```python
from build123d import *

# Parameters (mm, degrees)
SKETCH_1_W          = 100
SKETCH_1_H          = 50
EXTRUDE_1_DEPTH     = 10
SKETCH_2_R          = 5
EXTRUDE_2_DEPTH     = 10
HOLE_WIZARD_1_D     = 8.647
HOLE_WIZARD_1_DEPTH = 26.2
HOLE_WIZARD_1_TIP   = 2.597820886
FILLET_3_R          = 1
CHAMFER_2_SIZE      = 1
CHAMFER_3_SIZE      = 0.5


with BuildPart() as part:
    # 草圖1 → 擠出1 (new body)
    with BuildSketch(Plane(origin=(0, 0, 0), x_dir=(-1, 0, 0), z_dir=(0, 1, 0))):
        Rectangle(SKETCH_1_W, SKETCH_1_H)
    extrude(amount=EXTRUDE_1_DEPTH)

    # 草圖2 → 擠出2 (cut)
    with BuildSketch(Plane(origin=(0, 10, 0), x_dir=(-1, 0, 0), z_dir=(0, 1, 0))):
        with Locations(Location((-30, -12.5, 0), (0, 0, 90))):
            Circle(SKETCH_2_R)
        with Locations(Location((-30, 12.5, 0), (0, 0, 90))):
            Circle(SKETCH_2_R)
    extrude(amount=-EXTRUDE_2_DEPTH, mode=Mode.SUBTRACT)

    # 孔1
    with Locations(Plane(origin=(0, 10, 0), x_dir=(1, 0, 0), z_dir=(0, 1, 0))):
        with Locations((-30, -12.5), (-30, 12.5)):
            Hole(HOLE_WIZARD_1_D / 2, depth=HOLE_WIZARD_1_DEPTH)
            with Locations((0, 0, -(HOLE_WIZARD_1_DEPTH + HOLE_WIZARD_1_TIP / 2))):  # 118° drill point
                Cone(0, HOLE_WIZARD_1_D / 2, HOLE_WIZARD_1_TIP, mode=Mode.SUBTRACT)

    # 圓角3
    fillet_3_edges = [part.edges().sort_by_distance(p)[0] for p in [
        (-50, 5, -25),
        (50, 5, -25),
        (50, 5, 25),
        (-50, 5, 25),
    ]]
    fillet(fillet_3_edges, radius=FILLET_3_R)

    # 倒角2
    chamfer_2_edges = [part.edges().sort_by_distance(p)[0] for p in [
        (0, 0, -25),
        (0, 10, -25),
        (-50, 0, 0),
        (50, 0, 0),
        (0, 0, 25),
        (-49.707106781, 0, 24.707106781),
        (-49.707106781, 0, -24.707106781),
        (49.707106781, 0, 24.707106781),
        (49.707106781, 0, -24.707106781),
        (50, 10, 0),
        (-50, 10, 0),
        (0, 10, 25),
        (-49.707106781, 10, 24.707106781),
        (-49.707106781, 10, -24.707106781),
        (49.707106781, 10, 24.707106781),
        (49.707106781, 10, -24.707106781),
    ]]
    chamfer(chamfer_2_edges, length=CHAMFER_2_SIZE)

    # 倒角3
    chamfer_3_edges = [part.edges().sort_by_distance(p)[0] for p in [
        (30, 10, -17.5),
        (30, 10, 7.5),
    ]]
    chamfer(chamfer_3_edges, length=CHAMFER_3_SIZE)


solid = part.part
```
Part model, mm, in its own coordinate system. Coordinates: 2 decimals unless noted, no trailing zeros. Order: outer loops, then holes, each group sorted by start corner. A loop starts at its lowest first (then second) coordinate and runs counter-clockwise, first axis right, second up. Notation, with made-up numbers: (-4.5, -36) -> (9.5, -36) arc R24 cw to (9.5, -23) -> close; hole circle Ø9 at (10, 23.25). An arc over 180 degrees is marked (long way). Put each result on its own line as item: value. Start each with the question number.
(1) Probe line 1 along Z through (x, y) = (-30, 6.25); line 2 along X through (y, z) = (2.5, 9); line 3 along Z through (x, y) = (32.5, 9.75). List the from-to ranges inside material, lowest first. Write a range as [from, to].
(2) Band-saw the part on A-A (z = 12.5). Give the cut face in (x, y), then the cut area to 3 significant figures.
(3) Band-saw the part on C-C (y = 6.5). Give the cut face in (x, z), then the cut area to 3 significant figures.
(4) Pin check, flat tips, straight feed: pin 1 Ø12 at (x, z) = (17.5, 10.5) entering from -Y; pin 2 Ø9 at (x, z) = (30, -12.5) entering from -Y. Stop position of each tip, or through.
(5) Mould opens along Z. For faces 1 (the face through (1, 5, -25)), 2 (the face through (25.564, 4.816, 14.807)), 3 (the face through (1, 10, 0)) say: pulls with the +Z half, pulls with the -Z half, needs draft (parallel to the pull), parting line crosses it, or undercut.
(6) Band-saw the part on D-D (x = -30). Give the cut face in (y, z), then the cut area to 3 significant figures.
(7) Band-saw the part on B-B (x = 30). Give the cut face in (y, z), then the cut area to 4 significant figures.
Determined:
1. line 1: z = [-25, -16.82], [-8.18, 8.18], [16.82, 25]
1. line 2: x = [-50, -32.54], [-27.46, 26.43], [33.57, 50]
1. line 3: z = [-24.25, -17.12], [-7.88, 7.88], [17.12, 24.25]
2. outline: (-50, 1) -> (-49, 0) -> (-34.32, 0) -> (-34.32, 10) -> (-49, 10) -> (-50, 9) -> close; (-25.68, 0) -> (25, 0) -> (25, 9.5) -> (24.5, 10) -> (-25.68, 10) -> close; (35, 0) -> (49, 0) -> (50, 1) -> (50, 9) -> (49, 10) -> (35.5, 10) -> (35, 9.5) -> close
2. area: 811 mm²
3. outline: (-50, -24) arc R1 ccw to (-49, -25) -> (49, -25) arc R1 ccw to (50, -24) -> (50, 24) arc R1 ccw to (49, 25) -> (-49, 25) arc R1 ccw to (-50, 24) -> close; hole circle Ø8.65 at (-30, -12.5); hole circle Ø8.65 at (-30, 12.5); hole circle Ø10 at (30, -12.5); hole circle Ø10 at (30, 12.5)
3. area: 4,720 mm²
4. pin 1: stops at y = 0
4. pin 2: passes through
5. face 1: pulls with the -Z half
5. face 2: undercut
5. face 3: needs draft
6. outline: (0, -24) -> (1, -25) -> (9, -25) -> (10, -24) -> (10, -16.82) -> (0, -16.82) -> close; (0, -8.18) -> (10, -8.18) -> (10, 8.18) -> (0, 8.18) -> close; (0, 16.82) -> (10, 16.82) -> (10, 24) -> (9, 25) -> (1, 25) -> (0, 24) -> close
6. area: 325 mm²
7. outline: (0, -24) -> (1, -25) -> (9, -25) -> (10, -24) -> (10, -18) -> (9.5, -17.5) -> (0, -17.5) -> close; (0, -7.5) -> (9.5, -7.5) -> (10, -7) -> (10, 7) -> (9.5, 7.5) -> (0, 7.5) -> close; (0, 17.5) -> (9.5, 17.5) -> (10, 18) -> (10, 24) -> (9, 25) -> (1, 25) -> (0, 24) -> close
7. area: 297.5 mm²
